```python
from build123d import *

# Parameters (mm, degrees)
SKETCH1_W           = 20
SKETCH1_H           = 20
BOSS_EXTRUDE1_DEPTH = 6
SKETCH2_W           = 24
SKETCH2_H           = 24
BOSS_EXTRUDE2_DEPTH = 1
SKETCH2_3_W         = 26
SKETCH2_3_H         = 26
SKETCH2_3_W_2       = 24
SKETCH2_3_H_2       = 24
BOSS_EXTRUDE3_DEPTH = 8
FILLET1_R           = 2
FILLET2_R           = 2


with BuildPart() as part:
    # Sketch1 → Boss-Extrude1 (new body)
    with BuildSketch(Plane(origin=(0, 0, 0), x_dir=(1, 0, 0), z_dir=(0, 1, 0))):
        Rectangle(SKETCH1_W, SKETCH1_H)
    extrude(amount=BOSS_EXTRUDE1_DEPTH)

    # Sketch2 → Boss-Extrude2 (add)
    with BuildSketch(Plane(origin=(0, 0, 0), x_dir=(1, 0, 0), z_dir=(0, 1, 0))):
        Rectangle(SKETCH2_W, SKETCH2_H)
    extrude(amount=BOSS_EXTRUDE2_DEPTH)

    # Sketch2<3> → Boss-Extrude3 (add)
    with BuildSketch(Plane(origin=(0, 0, 0), x_dir=(1, 0, 0), z_dir=(0, 1, 0))):
        Rectangle(SKETCH2_3_W, SKETCH2_3_H)
        Rectangle(SKETCH2_3_W_2, SKETCH2_3_H_2, mode=Mode.SUBTRACT)
    extrude(amount=BOSS_EXTRUDE3_DEPTH)

    # Fillet1
    fillet1_edges = [part.edges().sort_by_distance(p)[0] for p in [
        (10, 3.5, 10),
        (-10, 3.5, 10),
        (-10, 3.5, -10),
        (10, 3.5, -10),
    ]]
    fillet(fillet1_edges, radius=FILLET1_R)

    # Fillet2
    fillet2_edges = [part.edges().sort_by_distance(p)[0] for p in [
        (12, 4.5, -12),
        (-12, 4.5, -12),
        (-12, 4.5, 12),
        (12, 4.5, 12),
    ]]
    fillet(fillet2_edges, radius=FILLET2_R)


solid = part.part
```
Model file for the job. Use its own axes, mm. A direction names the side the tool comes from. Coordinates: 2 decimals unless noted, no trailing zeros. Order: outer loops, then holes, each group sorted by start corner. A loop starts at its lowest first (then second) coordinate and runs counter-clockwise, first axis right, second up. Notation, with made-up numbers: (28, 69.5) -> (66, 69.5) arc R19 cw to (66, 77.5) -> close; hole circle Ø1 at (3.5, -2). An arc over 180 degrees is marked (long way). Answer as a JSON object with one key per item and string values. Group by question number.
1) Cut at C-C, the plane x = 2.25. Write the cut outline in (y, z), then the cut area to 3 significant figures.
2) Cut at A-A, the plane y = 5.25. Write the cut outline in (x, z), then the cut area to 3 significant figures.
3) Drill centre lines: L1, parallel to Z at x = -6.75, y = 2.25; L2, parallel to X at y = 6.5, z = 8.25. Where is each one in solid material? Low to high.
4) Which spindle directions (+Z, -Z, +X, -X, +Y, -Y) get a long thin tool onto all of the face, cutting with end or side? Do faces 5 (the face through (0, 3, 10)), 6 (the face through (0, 4, -13)). Say none if no direction does.
5) Flat gauge pin, fed straight in: pin 1 (5 mm diameter, centred on x = -8.5, z = 3, fed in from +Y). Where does the tip first touch, or does it go through?
6) Pull direction X, two halves, no side cores. Call faces 1 (the face through (10.5, 1, -0.2)), 2 (the face through (-0.1, 8, -12.6)), 3 (the face through (13, 4, 0)), 4 (the face through (-11.43, 4.55, -11.4)): +X half, -X half, draft (parallel to the pull), parting line (faces both ways), or undercut.
7) Cut at B-B, the plane z = 1. Write the cut outline in (x, y).
8) Cut at D-D, the plane x = 11. Write the cut outline in (y, z).
Check values:
{
 "1": {"outline": "(0, -13) -> (8, -13) -> (8, -12) -> (1, -12) -> (1, -10) -> (6, -10) -> (6, 10) -> (1, 10) -> (1, 12) -> (8, 12) -> (8, 13) -> (0, 13) -> close", "area": "140 mm²"},
 "2": {"outline": "(-13, -13) -> (13, -13) -> (13, 13) -> (-13, 13) -> close; (-10, -8) arc R2 ccw to (-8, -10) -> (8, -10) arc R2 ccw to (10, -8) -> (10, 8) arc R2 ccw to (8, 10) -> (-8, 10) arc R2 ccw to (-10, 8) -> close; hole (-12, -10) arc R2 ccw to (-10, -12) -> (10, -12) arc R2 ccw to (12, -10) -> (12, 10) arc R2 ccw to (10, 12) -> (-10, 12) arc R2 ccw to (-12, 10) -> close", "area": "500 mm²"},
 "3": {"L1": "z = -13 to -12, -10 to 10, 12 to 13", "L2": "x = -13 to -12, 12 to 13"},
 "4": {"face 5": "+Y", "face 6": "-Z, +X, -X, +Y, -Y"},
 "5": {"pin 1": "stops at y = 6"},
 "6": {"face 1": "undercut", "face 2": "draft", "face 3": "+X half", "face 4": "undercut"},
 "7": {"outline": "(-13, 0) -> (13, 0) -> (13, 8) -> (12, 8) -> (12, 1) -> (10, 1) -> (10, 6) -> (-10, 6) -> (-10, 1) -> (-12, 1) -> (-12, 8) -> (-13, 8) -> close"},
 "8": {"outline": "(0, -13) -> (8, -13) -> (8, -11.73) -> (1, -11.73) -> (1, 11.73) -> (8, 11.73) -> (8, 13) -> (0, 13) -> close"}
}
